Geometry: see drawing. Coordinates: mm, zero at the bounding-box minimum. A direction names the side the tool comes from. Round coordinates to 2 decimals unless told otherwise and drop trailing zeros. Write each loop counter-clockwise with the first axis right and the second up, starting at its lowest first coordinate (ties: lowest second). Pieces come first, ordered by that corner, then holes. Notation, with made-up numbers: M -11,-32.75 L 6,-32.75 A26 cw 6,-8.75 Z; hole C -1.75,9 d11. An arc over 180 degrees is marked long. Write each question's results on one line, items separated by ' | '. Start each with the question number.
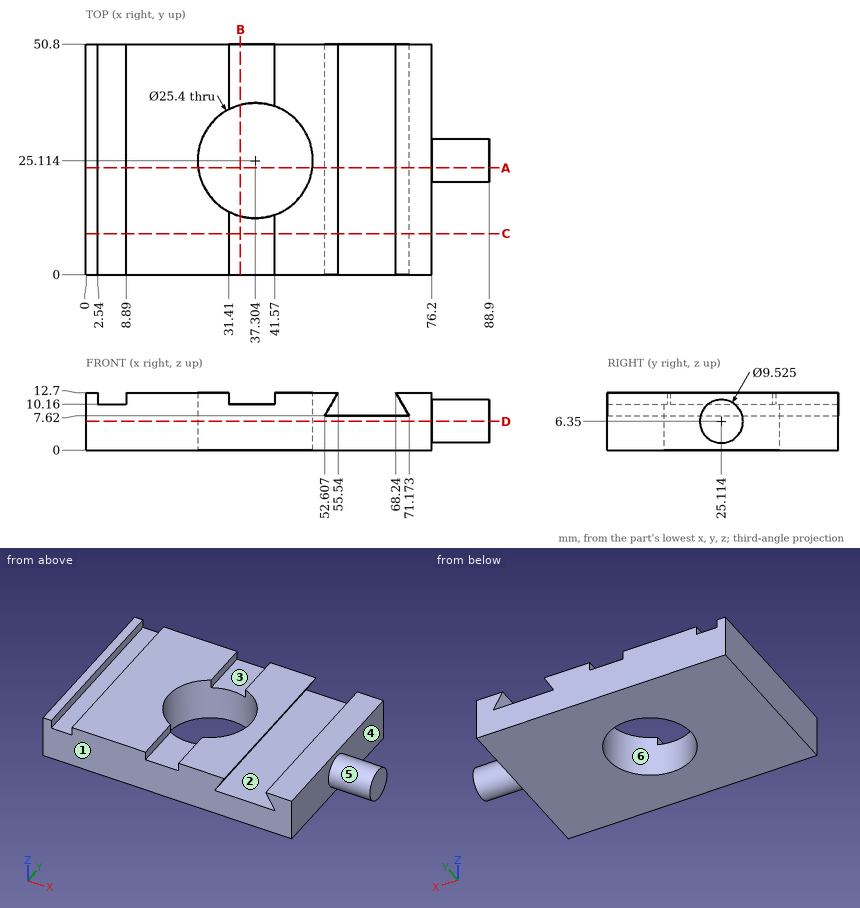
1. Cut plane D-D on z = 6.35. Output: boundary loops of the cut face in (x, y).
2. Cut plane C-C on y = 9. Output: boundary loops of the cut face in (x, z).
3. Cut plane A-A on y = 23.5. Output: boundary loops of the cut face in (x, z), and give its area (3 significant figures).
4. Draft query along Y for the marked faces 4, 5 and 6. Return one class per face: +Y half, -Y half, draft (parallel to the pull), parting line (faces both ways), or undercut.
5. Access query for the marked faces 1, 2 and 3. Directions: +Z, -Z, +X, -X, +Y, -Y. A direction counts if a zero-diameter tool reaches every point of the face in a straight line with its end or side. Return the directions, or none.
6. Contact query for flat-ended pins moving along their axis: P1, Ø2, axis at y = 43.5, z = 11, coming from the +X side; P2, Ø5, axis at x = 36, y = 42, coming from the +Z side. Output: stop coordinate, or through.
7. Cut plane B-B on x = 34. Output: boundary loops of the cut face in (y, z), and give its area (3 significant figures).
8. Line query: L1, parallel to Z at x = 56, y = 42.5; L2, parallel to Y at x = 38, z = 9.75 (1 decimal); L3, parallel to Z at x = 5, y = 16. Output: solid intervals per line, ascending. Write a range as from..to.
Answers follow:
1) outline: M 0,0 L 76.2,0 L 76.2,20.35 L 88.9,20.35 L 88.9,29.88 L 76.2,29.88 L 76.2,50.8 L 0,50.8 Z; hole C 37.3,25.11 d25.4
2) outline: M 0,0 L 76.2,0 L 76.2,12.7 L 68.24,12.7 L 71.17,7.62 L 52.61,7.62 L 55.54,12.7 L 41.57,12.7 L 41.57,10.16 L 31.41,10.16 L 31.41,12.7 L 8.89,12.7 L 8.89,10.16 L 2.54,10.16 L 2.54,12.7 L 0,12.7 Z
3) outline: M 0,0 L 24.71,0 L 24.71,12.7 L 8.89,12.7 L 8.89,10.16 L 2.54,10.16 L 2.54,12.7 L 0,12.7 Z; M 49.9,0 L 76.2,0 L 76.2,1.87 L 88.9,1.87 L 88.9,10.83 L 76.2,10.83 L 76.2,12.7 L 68.24,12.7 L 71.17,7.62 L 52.61,7.62 L 55.54,12.7 L 49.9,12.7 Z | area: 666 mm2
4) face 4: draft | face 5: parting line | face 6: undercut
5) face 1: +Z, -Z, +X, -X, -Y | face 2: +Y, -Y | face 3: +Z, +Y, -Y
6) P1: stops at x = 76.2 | P2: stops at z = 10.16
7) outline: M 0,0 L 12.85,0 L 12.85,10.16 L 0,10.16 Z; M 37.38,0 L 50.8,0 L 50.8,10.16 L 37.38,10.16 Z | area: 267 mm2
8) L1: z = 0..7.62 | L2: y = 0..12.4, 37.8..50.8 | L3: z = 0..10.16
